The listing builds one solid part. Answer for the finished solid, in the listing's coordinates (mm). A direction names the side the tool comes from. Coordinates: 2 decimals unless noted, no trailing zeros. Write each loop counter-clockwise with the first axis right and the second up, starting at its lowest first coordinate (ties: lowest second). Pieces come first, ordered by that corner, then holes. Notation, with made-up numbers: M 26.25,20.5 L 39.25,20.5 A11 cw 39.25,27.5 Z; hole C 24,53.25 d10. An arc over 180 degrees is marked long. Put each result on its own line as item: value. Start each with the question number.
```python
from build123d import *

# Parameters (mm, degrees)
SKETCH3_W                 = 140
SKETCH3_H                 = 140
BOSS_EXTRUDE1_DEPTH       = 5
CUT_EXTRUDE1_DEPTH        = 5
CIRPATTERN1_COUNT         = 4
CUT_EXTRUDE2_REACH        = 101.121
SKETCH7_R                 = 11
CIRPATTERN2_COUNT         = 4
CHAMFER1_SIZE             = 5
F_3_0MM_DOWEL_HOLE2_D     = 2.8
F_3_0MM_DOWEL_HOLE2_DEPTH = 10
MIRROR3_COPY_1_D          = 2.8
MIRROR3_COPY_1_DEPTH      = 10


with BuildPart() as part:
    # Sketch3 → Boss-Extrude1 (new body)
    with BuildSketch(Plane.XY):
        Rectangle(SKETCH3_W, SKETCH3_H)
    extrude(amount=BOSS_EXTRUDE1_DEPTH)

    # Sketch4 → Cut-Extrude1 (cut)
    with BuildSketch(Plane.XY.offset(5)):
        with BuildLine():
            Line((7.583144073, 14.654211885), (52.928932188, 60))
            Line((52.928932188, 60), (-54.688394727, 60))
            Line((-54.688394727, 60), (-7.80758307, 14.53587447))
            ThreePointArc((-7.80758307, 14.53587447), (-0.126862728, 16.499512291), (7.583144073, 14.654211885))
        make_face()
    cut_extrude1 = extrude(amount=-CUT_EXTRUDE1_DEPTH, mode=Mode.SUBTRACT)

    # CirPattern1: Cut-Extrude1 ×4 about axis
    cirpattern1_axis = Axis((0, 0, 0), (0, 0, 1))
    for i in range(1, CIRPATTERN1_COUNT):
        add(cut_extrude1.rotate(cirpattern1_axis, i * 360 / CIRPATTERN1_COUNT), mode=Mode.SUBTRACT)

    # Sketch7 → Cut-Extrude2 (cut, up to next)
    with BuildSketch(Plane.XY.offset(5), mode=Mode.PRIVATE) as cut_extrude2_sk1:
        Circle(SKETCH7_R)
    cut_extrude2_tool1 = extrude(cut_extrude2_sk1.sketch, amount=-CUT_EXTRUDE2_REACH, mode=Mode.PRIVATE) & part.part
    add(cut_extrude2_tool1.solids().sort_by_distance((0, 0, 5))[0], mode=Mode.SUBTRACT)

    # Sketch9 → Ø1.8 (1.8) Diameter Hole1 (revolve, cut)
    with BuildSketch(Plane(origin=(11.313708499, -11.313708499, 5), x_dir=(0, -1, 0), z_dir=(1, 0, 0))):
        Polygon((0, 0), (0, 6.540774557), (0.9, 6), (0.9, 0), align=None)
    f_1_8_1_8_diameter_hole1 = revolve(axis=Axis((11.313708499, -11.313708499, 11.35), (0, 0, -1)), mode=Mode.SUBTRACT)

    # CirPattern2: Ø1.8 (1.8) Diameter Hole1 ×4 about axis
    cirpattern2_axis = Axis((0, 0, 0), (0, 0, 1))
    for i in range(1, CIRPATTERN2_COUNT):
        add(f_1_8_1_8_diameter_hole1.rotate(cirpattern2_axis, i * 360 / CIRPATTERN2_COUNT), mode=Mode.SUBTRACT)

    # Chamfer1
    chamfer1_edges = [part.edges().sort_by_distance(p)[0] for p in [
        (0, 70, 5),
        (0, -70, 5),
    ]]
    chamfer(chamfer1_edges, length=CHAMFER1_SIZE - 0.0001)  # a hair under: the kernel refuses the full size

    # Sketch12 → Ø3.0mm Dowel Hole1 (revolve, cut)
    with BuildSketch(Plane(origin=(-70, 63, 2.5), x_dir=(0, 0, 1), z_dir=(0, 1, 0))):
        Polygon((0, 0), (0, 10.841204867), (1.4, 10), (1.4, 0), align=None)
    f_3_0mm_dowel_hole1 = revolve(axis=Axis((-76.35, 63, 2.5), (1, 0, 0)), mode=Mode.SUBTRACT)

    # Mirror1: Ø3.0mm Dowel Hole1 across plane
    add(f_3_0mm_dowel_hole1.mirror(Plane.ZX), mode=Mode.SUBTRACT)

    # Ø3.0mm Dowel Hole2
    with Locations(Plane(origin=(55, 67.5, 2.5), x_dir=(0, -0.707106781187, 0.707106781187), z_dir=(0, 0.707106781187, 0.707106781187))):
        with Locations((0, 0)):
            f_3_0mm_dowel_hole2 = Hole(F_3_0MM_DOWEL_HOLE2_D / 2, depth=F_3_0MM_DOWEL_HOLE2_DEPTH)

    # Mirror2: Ø3.0mm Dowel Hole2 across plane
    add(f_3_0mm_dowel_hole2.mirror(Plane(origin=(0, 0, 0), x_dir=(0, 0, 1), z_dir=(1, 0, 0))), mode=Mode.SUBTRACT)

    # Mirror3: Ø3.0mm Dowel Hole2 across plane
    add(f_3_0mm_dowel_hole2.mirror(Plane.ZX), mode=Mode.SUBTRACT)

    # Mirror3 copy 1
    with Locations(Plane(origin=(-55, -67.5, 2.5), x_dir=(0, 0.707106781187, 0.707106781187), z_dir=(0, -0.707106781187, 0.707106781187))):
        with Locations((0, 0)):
            Hole(MIRROR3_COPY_1_D / 2, depth=MIRROR3_COPY_1_DEPTH)


solid = part.part
```
1) A cutting plane is placed at C-C on y = 39.5. Write down the section's boundary in (x, z), then the cut area to 3 significant figures.
2) A cutting plane is placed at B-B on y = 0. Write down the section's boundary in (x, z).
3) Straight lines are drawn through the part: probe 1 along Y at (x, z) = (-39.5, 0.65); probe 2 along Y at (x, z) = (-41, 4); probe 3 along X at (y, z) = (11.5, 1.45). For each, find the intervals that lie inside material, in ascending order.
4) For faces 1 (the face through (-70, -1, 2)), 2 (the face through (60, 0, 3)), determine the directions among +Z, -Z, +X, -X, +Y, -Y from which every point of the face is accessible in a straight line to the end or side of a thin tool.
5) A cutting plane is placed at A-A on x = 0. State how many separate pieces and enclosed holes the cut face has, then the cut area to 3 significant figures.
6) Determine the mould class of faces 3 (the face through (70, -1, 2)), 4 (the face through (-55.06, -65.09, 2.07)), 5 (the face through (-1, -67, 3)) for opening direction X: +X half, -X half, draft (parallel to the pull), parting line (faces both ways), or undercut.
7) Given pin 1 Ø1.5 at (x, z) = (-2, 4.5) entering from -Y, flat-ended and moving along its own axis, determine where the tip first touches the part or whether it passes through.
Answers follow:
1. outline: M -70,0 L -60,0 L -60,5 L -70,5 Z; M -46.57,0 L -33.55,0 L -33.55,5 L -46.57,5 Z; M 32.43,0 L 45.27,0 L 45.27,5 L 32.43,5 Z; M 60,0 L 70,0 L 70,5 L 60,5 Z
1. area: 229 mm²
2. outline: M -70,0 L -60,0 L -60,5 L -70,5 Z; M -16.5,0 L -11,0 L -11,5 L -16.5,5 Z; M 11,0 L 16.5,0 L 16.5,5 L 11,5 Z; M 60,0 L 70,0 L 70,5 L 60,5 Z
3. probe 1: y = -69.35 to -60, -46.57 to -33.55, 32.43 to 45.27, 60 to 69.35
3. probe 2: y = -66 to -60, -48.07 to -35.1, 33.93 to 46.73, 60 to 66
3. probe 3: x = -70 to -60, -18.57 to -12.19, -10.43 to 10.43, 12.19 to 18.12, 60 to 70
4. face 1: +Z, -Z, -X, +Y, -Y
4. face 2: +Z, -Z
5. separate pieces: 4
5. enclosed holes: 0
5. area: 130 mm²
6. face 3: +X half
6. face 4: undercut
6. face 5: draft
7. pin 1: stops at y = -66.25
